For this review, take the finished solid that the model builds, in its own axes (mm). A direction names the side the tool comes from. Round coordinates to 2 decimals unless told otherwise and drop trailing zeros. Order: outer loops, then holes, each group sorted by start corner. A loop starts at its lowest first (then second) coordinate and runs counter-clockwise, first axis right, second up. Notation, with made-up numbers: M 59,40 L 72,40 A30 cw 72,78 Z; hole C 2.25,72.25 d4. An arc over 180 degrees is marked long. Use a Markdown table: item, result.
from build123d import *

# Parameters (mm, degrees)
BOSS_EXTRUDE1_DEPTH = 38.1
SKETCH2_R           = 12.065
CUT_EXTRUDE1_DEPTH  = 15.24
SKETCH3_R           = 12.065
CUT_EXTRUDE2_DEPTH  = 15.24
CUT_EXTRUDE3_DEPTH  = 38.1


with BuildPart() as part:
    # Sketch1 → Boss-Extrude1 (new body)
    with BuildSketch(Plane(origin=(0, 0, 0), x_dir=(1, 0, 0), z_dir=(0, 1, 0))):
        Polygon((0, 0), (113.579665808, 0), (124.068494586, -14.211767965), (154.723601267, 8.412874228), (127.782832904, 35.353642591), (-14.203167096, 35.353642591), (-41.143935459, 8.412874228), (-10.488828778, -14.211767965), align=None)
    extrude(amount=BOSS_EXTRUDE1_DEPTH)

    # Sketch2 → Cut-Extrude1 (cut)
    with BuildSketch(Plane(origin=(-10.488828778, 0, 14.211767965), x_dir=(0.8045959758833214, 0, 0.5938226297408727), z_dir=(-0.5938226297408727, 0, 0.8045959758833214))):
        with Locations((-19.05, 19.05)):
            Circle(SKETCH2_R)
    extrude(amount=-CUT_EXTRUDE1_DEPTH, mode=Mode.SUBTRACT)

    # Sketch3 → Cut-Extrude2 (cut)
    with BuildSketch(Plane(origin=(50.539894278, 0, 68.478689631), x_dir=(0.8045959758833213, 0, -0.5938226297408729), z_dir=(0.5938226297408729, 0, 0.8045959758833213))):
        with Locations((110.435742051, 19.05)):
            Circle(SKETCH3_R)
    extrude(amount=-CUT_EXTRUDE2_DEPTH, mode=Mode.SUBTRACT)

    # Sketch5 → Cut-Extrude3 (cut)
    with BuildSketch(Plane(origin=(0, 38.1, 0), x_dir=(1, 0, 0), z_dir=(0, 1, 0))):
        Polygon((4.151555437, 17.676821295), (20.32, 30.376821295), (20.32, 4.976821295), align=None)
        Polygon((45.384535252, 30.376821295), (45.384535252, 4.976821295), (56.789832904, 13.935461665), (68.195130556, 4.976821295), (68.195130556, 30.376821295), (56.789832904, 21.418180926), align=None)
        Polygon((93.259665808, 30.376821295), (93.259665808, 4.976821295), (109.428110371, 17.676821295), align=None)
    extrude(amount=-CUT_EXTRUDE3_DEPTH, mode=Mode.SUBTRACT)


solid = part.part
Q1. Clearance check with flat-ended pins moving along their axes: pin 1 (20.5 mm diameter, centred on y = 11, z = -18, fed in from +X); pin 2 (2 mm diameter, centred on x = -17.5, y = 20.5, fed in from -Z); pin 3 (8 mm diameter, centred on y = 8.5, z = -22, fed in from +X). State where each tip first meets the part, or that it passes through.
Determined:
| item | result |
|---|---|
| pin 1 | stops at x = 154.72 |
| pin 2 | stops at z = -33.06 |
| pin 3 | stops at x = 145.14 |
Q2. Add section C-C (y = 22.5). Write out the cut boundary in (x, z), then the cut area to 3 significant figures.
Determined:
| item | result |
|---|---|
| outline | M -41.14,-8.41 L -14.2,-35.35 L 127.78,-35.35 L 154.72,-8.41 L 148.7,-3.97 L 139.65,-16.23 L 121.04,-2.5 L 130.09,9.76 L 124.07,14.21 L 113.58,0 L 0,0 L -10.49,14.21 L -16.51,9.76 L -7.46,-2.5 L -26.07,-16.23 L -35.12,-3.97 Z; hole M 4.15,-17.68 L 20.32,-30.38 L 20.32,-4.98 Z; hole M 45.38,-30.38 L 56.79,-21.42 L 68.2,-30.38 L 68.2,-4.98 L 56.79,-13.94 L 45.38,-4.98 Z; hole M 93.26,-30.38 L 109.43,-17.68 L 93.26,-4.98 Z |
| area | 5,040 mm^2 |
Q3. Machinability: for faces 1 (the flat face through (130.21, 19.22, -9.26)), 2 (the flat face through (55, 38.1, -11)), 3 (the flat face through (45.385, 19, -18)), 4 (the flat face through (58, 19, -35.354)), 5 (the flat face through (-5.32, 18.78, 7.21)), which of the approach directions +Z, -Z, +X, -X, +Y, -Y give a long, thin tool a straight path to every point of the face, cutting with its end or side? Answer none if there is none.
Determined:
| item | result |
|---|---|
| face 1 | none |
| face 2 | +Z, -Z, +X, -X, +Y |
| face 3 | +Y, -Y |
| face 4 | -Z, +X, -X, +Y, -Y |
| face 5 | +Z, +Y, -Y |
Q4. Wall thickness on line 1 along X through (y, z) = (28, -3.5); line 2 along Y through (x, z) = (127, -3); line 3 along Z through (x, y) = (87, 22): over which ranges is each line inside the solid? List them lowest first. Write a range as [from, to].
Determined:
| item | result |
|---|---|
| line 1 | x = [-34.49, -31.15], [-11.04, 124.62], [144.73, 148.07] |
| line 2 | y = [0, 8.87], [29.23, 38.1] |
| line 3 | z = [-35.35, 0] |
Q5. Add section A-A (y = 15). Write out the cut boundary in (x, z), then the cut area to 3 significant figures.
Determined:
| item | result |
|---|---|
| outline | M -41.14,-8.41 L -14.2,-35.35 L 127.78,-35.35 L 154.72,-8.41 L 148.54,-3.85 L 139.49,-16.11 L 121.2,-2.61 L 130.25,9.65 L 124.07,14.21 L 113.58,0 L 0,0 L -10.49,14.21 L -16.67,9.65 L -7.62,-2.61 L -25.91,-16.11 L -34.96,-3.85 Z; hole M 4.15,-17.68 L 20.32,-30.38 L 20.32,-4.98 Z; hole M 45.38,-30.38 L 56.79,-21.42 L 68.2,-30.38 L 68.2,-4.98 L 56.79,-13.94 L 45.38,-4.98 Z; hole M 93.26,-30.38 L 109.43,-17.68 L 93.26,-4.98 Z |
| area | 5,050 mm^2 |
Q6. Add section B-B (x = 91.5). Write out the cut boundary in (y, z).
Determined:
| item | result |
|---|---|
| outline | M 0,-35.35 L 38.1,-35.35 L 38.1,0 L 0,0 Z |
Q7. Draft analysis for pull direction X (two halves, no side actions). For faces 6 (the flat face through (132.369, 10.317, 8.086)), 7 (the cylindrical face through (-31.053, 19.58, -10.303)), 8 (the flat face through (-27.485, 18.783, -22.072)), state which applies: pulls with the +X half, pulls with the -X half, needs draft (parallel to the pull), parting line crosses it, or undercut.
Determined:
| item | result |
|---|---|
| face 6 | pulls with the +X half |
| face 7 | undercut |
| face 8 | pulls with the -X half |
